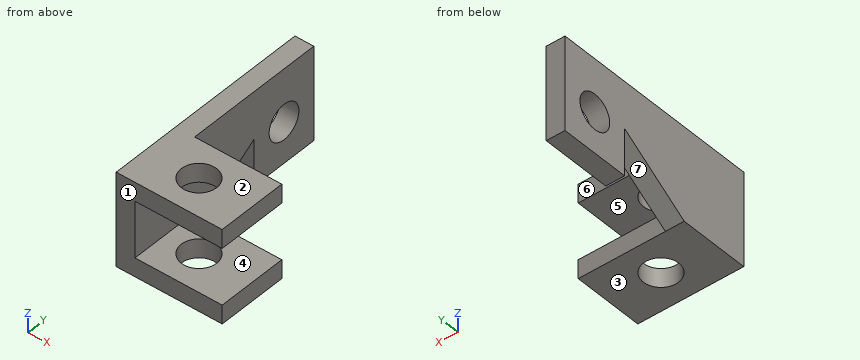
from build123d import *

# Parameters (mm, degrees)
F1_DEPTH = 203.2
F2_W     = 762
F2_H     = 203.2
F3_DEPTH = 939.8
F5_D     = 381
F7_D     = 381


with BuildPart() as f1:
    # F0 (on Right) → F1 (new body)
    with BuildSketch(Plane.YZ):
        Polygon((0, 1016), (0, 0), (762, 0), (1524, 508), (1524, 0), (2286, 0), (2286, 1016), align=None)
    extrude(amount=F1_DEPTH)

    # F2 (on face) → F3 (join)
    with BuildSketch(Plane.YZ.offset(203.2)):
        with Locations((381, 101.6)):
            Rectangle(F2_W, F2_H)
        with Locations((381, 914.4)):
            Rectangle(F2_W, F2_H)
    extrude(amount=F3_DEPTH)

    # F5 (through all)
    with Locations(Plane.XY.offset(1016)):
        with Locations((571.5, 381)):
            Hole(F5_D / 2)

    # F7 (through all)
    with Locations(Plane.YZ.offset(203.2)):
        with Locations((1905, 444.5)):
            Hole(F7_D / 2)


solid = f1.part
Geometry check sheet. Reference: the model listing, model coordinates, mm. Face numbers are marked on the shaded views. A direction names the side the tool comes from. Round coordinates to 2 decimals unless told otherwise and drop trailing zeros. Write each loop counter-clockwise with the first axis right and the second up, starting at its lowest first coordinate (ties: lowest second). Pieces come first, ordered by that corner, then holes.
Item 1: Material ranges on line 1 along Y through (x, z) = (571.5, 114); line 2 along Z through (x, y) = (318, 718.5); line 3 along Y through (x, z) = (120, 444), recorded low to high.
Determined:
line 1: y = 0 to 190.5, 571.5 to 762
line 2: z = 0 to 203.2, 812.8 to 1016
line 3: y = 0 to 1428, 1524 to 1714.5, 2095.5 to 2286
Item 2: Mould release check, pull along Z, two halves, no side actions. Record for the marked faces 1, 2, 3 and 4: +Z half, -Z half, draft (parallel to the pull), parting line (faces both ways), or undercut.
Determined:
face 1: draft
face 2: +Z half
face 3: -Z half
face 4: undercut
Item 3: Access from +Z, -Z, +X, -X, +Y, -Y to the whole of each face (thin tool, end or side, straight path). Record for the marked faces 5, 6 and 7.
Determined:
face 5: +X, +Y, -Y
face 6: +Z, -Z, +X, +Y
face 7: -Z, +X, -X
Item 4: Go/stop test with a flat-tipped pin: pin 1 Ø5 at (x, z) = (292.5, 193) entering from +Y. Record where the tip stops, or that it passes through.
Determined:
pin 1: stops at y = 762
Item 5: Section check B-B (x = 571.5). Record the boundary of the cut face in (y, z), plus the area to 3 significant figures.
Determined:
outline: (0, 0) - (190.5, 0) - (190.5, 203.2) - (0, 203.2) - close; (0, 812.8) - (190.5, 812.8) - (190.5, 1016) - (0, 1016) - close; (571.5, 0) - (762, 0) - (762, 203.2) - (571.5, 203.2) - close; (571.5, 812.8) - (762, 812.8) - (762, 1016) - (571.5, 1016) - close
area: 155,000 mm2
Item 6: Section check A-A (z = 67). Record the boundary of the cut face in (x, y), plus the area to 3 significant figures.
Determined:
outline: (0, 0) - (1143, 0) - (1143, 762) - (203.2, 762) - (203.2, 862.5) - (0, 862.5) - close; (0, 1524) - (203.2, 1524) - (203.2, 2286) - (0, 2286) - close; hole circle Ø381 at (571.5, 381)
area: 932,000 mm2
Item 7: Section check C-C (z = 444.5). Record the boundary of the cut face in (x, y).
Determined:
outline: (0, 0) - (203.2, 0) - (203.2, 1428.75) - (0, 1428.75) - close; (0, 1524) - (203.2, 1524) - (203.2, 1714.5) - (0, 1714.5) - close; (0, 2095.5) - (203.2, 2095.5) - (203.2, 2286) - (0, 2286) - close
Item 8: Section check D-D (y = 1905). Record the boundary of the cut face in (x, z).
Determined:
outline: (0, 0) - (203.2, 0) - (203.2, 254) - (0, 254) - close; (0, 635) - (203.2, 635) - (203.2, 1016) - (0, 1016) - close
